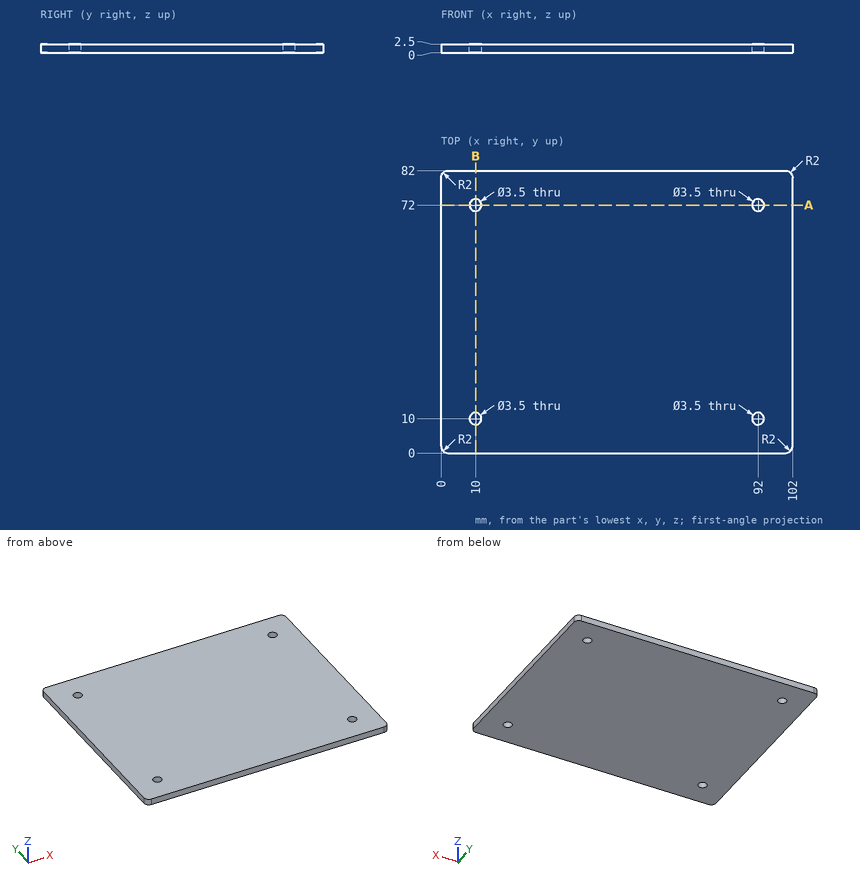
Geometry: see drawing. Coordinates: mm, zero at the bounding-box minimum. Coordinates: 2 decimals unless noted, no trailing zeros. Order: outer loops, then holes, each group sorted by start corner. A loop starts at its lowest first (then second) coordinate and runs counter-clockwise, first axis right, second up. Notation, with made-up numbers: M 41,4.5 L 76,4.5 A12 cw 76,10.5 Z; hole C -3,84 d4. An arc over 180 degrees is marked long. Write each question's results on one line, items separated by ' | '. Start each with the question number.
1) Section query B-B (x = 10). Return the cut outline in (y, z), plus the area to 4 significant figures.
2) Section query A-A (y = 72). Return the cut outline in (x, z).
3) Line query: line 1 (Y direction, x = 92, z = 1.5); line 2 (X direction, y = 72, z = 1.6). Output: solid intervals per line, ascending. Write a range as from..to.
Answers:
1) outline: M 0,0 L 8.25,0 L 8.25,2.5 L 0,2.5 Z; M 11.75,0 L 70.25,0 L 70.25,2.5 L 11.75,2.5 Z; M 73.75,0 L 82,0 L 82,2.5 L 73.75,2.5 Z | area: 187.5 mm^2
2) outline: M 0,0 L 8.25,0 L 8.25,2.5 L 0,2.5 Z; M 11.75,0 L 90.25,0 L 90.25,2.5 L 11.75,2.5 Z; M 93.75,0 L 102,0 L 102,2.5 L 93.75,2.5 Z
3) line 1: y = 0..8.25, 11.75..70.25, 73.75..82 | line 2: x = 0..8.25, 11.75..90.25, 93.75..102
